```python
from build123d import *

# Parameters (mm, degrees)
SKETCH3_W           = 52.07
SKETCH3_H           = 38.1
BOSS_EXTRUDE2_DEPTH = 3.81
SKETCH4_W           = 19.05
SKETCH4_H           = 12.7
CUT_EXTRUDE1_DEPTH  = 65.632894102
SKETCH6_R           = 1.651
CUT_EXTRUDE2_DEPTH  = 5.08
CUT_EXTRUDE3_START  = -5.08
SKETCH8_R           = 1.651
CUT_EXTRUDE3_DEPTH  = 5.08


with BuildPart() as part:
    # Sketch3 → Boss-Extrude2 (new body)
    with BuildSketch(Plane.XY):
        with Locations((26.035, 19.05)):
            Rectangle(SKETCH3_W, SKETCH3_H)
    extrude(amount=BOSS_EXTRUDE2_DEPTH)

    # Sketch4 → Cut-Extrude1 (cut, through all)
    with BuildSketch(Plane.XY.offset(3.81)):
        with Locations((26.035, 6.35)):
            Rectangle(SKETCH4_W, SKETCH4_H)
    extrude(amount=-CUT_EXTRUDE1_DEPTH, mode=Mode.SUBTRACT)

    # Sketch6 → Cut-Extrude2 (cut)
    with BuildSketch(Plane.XZ):
        with Locations(Location((8.255, 1.905, 0), (0, 0, 270))):
            Circle(SKETCH6_R)
        with Locations(Location((43.815, 1.905, 0), (0, 0, 270))):
            Circle(SKETCH6_R)
    extrude(amount=-CUT_EXTRUDE2_DEPTH, mode=Mode.SUBTRACT)

    # Sketch8 → Cut-Extrude3 (cut)
    with BuildSketch(Plane(origin=(0, 38.1, 0), x_dir=(1, 0, 0), z_dir=(0, 1, 0)).offset(CUT_EXTRUDE3_START)):
        with Locations(Location((8.255, -1.905, 0), (0, 0, 90))):
            Circle(SKETCH8_R)
        with Locations(Location((43.815, -1.905, 0), (0, 0, 90))):
            Circle(SKETCH8_R)
    extrude(amount=CUT_EXTRUDE3_DEPTH, mode=Mode.SUBTRACT)


solid = part.part
```
Design review of the part built by this model. Coordinates are the model's own, in mm. A direction names the side the tool comes from. Round coordinates to 2 decimals unless told otherwise and drop trailing zeros. Order: outer loops, then holes, each group sorted by start corner. A loop starts at its lowest first (then second) coordinate and runs counter-clockwise, first axis right, second up. Notation, with made-up numbers: (1.25, -4.5) - (10.25, -4.5) arc R27 ccw to (10.25, 11.5) - close; hole circle Ø10 at (-8, 30). An arc over 180 degrees is marked (long way). One line per question, with ' | ' between items.
Item 1: For P1, Ø1, axis at x = 43.5, z = 2, coming from the +Y side, flat-tipped, find the tip position at first contact; note if it passes through.
Checks:
P1: y = 33.02
Item 2: Machinability: for faces 1 (the face through (26, 12.7, 2)), 2 (the face through (45.427, 35.524, 2.263)), 3 (the face through (6, 0, 2)), 4 (the face through (8, 5.08, 2)), which of the approach directions +Z, -Z, +X, -X, +Y, -Y give a long, thin tool a straight path to every point of the face, cutting with its end or side? Answer none if there is none.
Checks:
face 1: +Z, -Z, -Y | face 2: +Y | face 3: +Z, -Z, +X, -X, -Y | face 4: -Y
Item 3: Wall thickness on line 1 (X direction, y = 9.5, z = 3.1); line 2 (Y direction, x = 28, z = 1.1); line 3 (X direction, y = 34.5, z = 3.05): over which ranges is each line inside the solid? List them lowest first. Write a range as [from, to].
Checks:
line 1: [0, 16.51], [35.56, 52.07] | line 2: [12.7, 38.1] | line 3: [0, 7.07], [9.44, 42.63], [45, 52.07]
Item 4: Take a section at B-B, the plane z = 1.3. Write out the cut boundary in (x, y).
Checks:
outline: (0, 0) - (6.72, 0) - (6.72, 5.08) - (9.79, 5.08) - (9.79, 0) - (16.51, 0) - (16.51, 12.7) - (35.56, 12.7) - (35.56, 0) - (42.28, 0) - (42.28, 5.08) - (45.35, 5.08) - (45.35, 0) - (52.07, 0) - (52.07, 38.1) - (45.35, 38.1) - (45.35, 33.02) - (42.28, 33.02) - (42.28, 38.1) - (9.79, 38.1) - (9.79, 33.02) - (6.72, 33.02) - (6.72, 38.1) - (0, 38.1) - close
Item 5: Take a section at A-A, the plane y = 11.5. Write out the cut boundary in (x, z), then the cut area to 3 significant figures.
Checks:
outline: (0, 0) - (16.51, 0) - (16.51, 3.81) - (0, 3.81) - close; (35.56, 0) - (52.07, 0) - (52.07, 3.81) - (35.56, 3.81) - close | area: 126 mm²
Item 6: Take a section at C-C, the plane x = 19. Write out the cut boundary in (y, z).
Checks:
outline: (12.7, 0) - (38.1, 0) - (38.1, 3.81) - (12.7, 3.81) - close
Item 7: Draft analysis for pull direction Z (two halves, no side actions). For faces 5 (the face through (26, 19, 0)), 6 (the face through (9.89, 2.5, 2.12)), 7 (the face through (16.51, 6, 2)), state which applies: +Z half, -Z half, draft (parallel to the pull), parting line (faces both ways), or undercut.
Checks:
face 5: -Z half | face 6: undercut | face 7: draft
